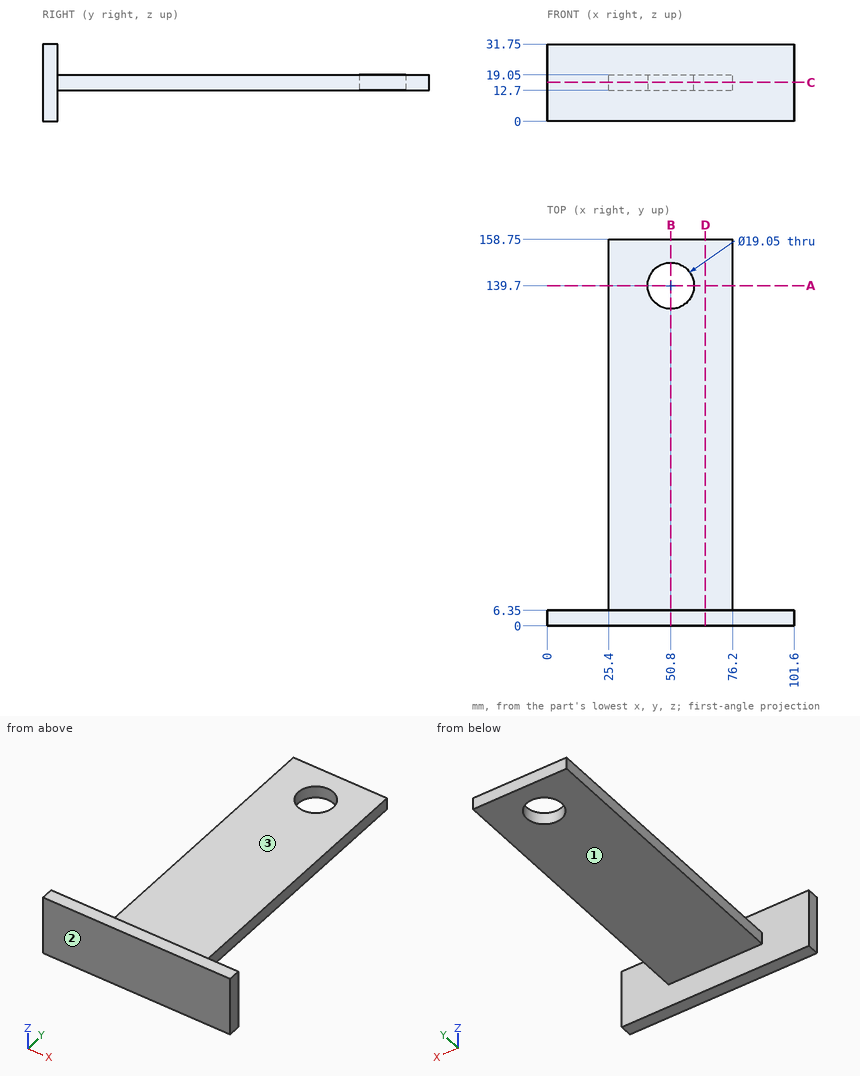
Source: three-view drawing plus pictorial views. Frame: mm from the lowest corner of the part. A direction names the side the tool comes from. Round coordinates to 2 decimals unless told otherwise and drop trailing zeros. Order: outer loops, then holes, each group sorted by start corner. A loop starts at its lowest first (then second) coordinate and runs counter-clockwise, first axis right, second up. Notation, with made-up numbers: (11, 44) -> (70, 44) arc R19 ccw to (70, 63) -> close; hole circle Ø6 at (26.5, -9.5). An arc over 180 degrees is marked (long way). Use CSV: the item, a comma, the result in double quotes. Start each with the question number.
1) Section C-C (z = 16). Return the cut outline in (x, y) (3 decimals).
2) Set-up query: the marked faces 1, 2 and 3. Return all of +Z, -Z, +X, -X, +Y, -Y with unobstructed straight access to the full face (end or side cutting, diameter ignored); none if empty.
3) Section B-B (x = 50.8). Return the cut outline in (y, z) (3 decimals).
4) Section A-A (y = 139.7). Return the cut outline in (x, z) (3 decimals), and give its area (3 significant figures).
5) Section D-D (x = 65). Return the cut outline in (y, z), and give its area (3 significant figures).
6) Material intervals for line 1 along Y through (x, z) = (50, 17); line 2 along X through (y, z) = (139.7, 17.75) (3 decimals); line 3 along Y through (x, z) = (20, 2.5), sorted ascending. Write a range as from..to.
7) First-contact query: pin 1 Ø6 at (x, y) = (63.5, 104) entering from +Z; pin 2 Ø3 at (y, z) = (84, 16) entering from +X; pin 3 Ø5 at (x, y) = (24.5, 117.5) entering from -Z; pin 4 Ø15 at (x, y) = (50.8, 139.7) entering from -Z. Flat tips, straight axial feed; report the tip coordinate or a pass-through.
Returned:
1,outline,"(0, 0) -> (101.6, 0) -> (101.6, 6.35) -> (76.2, 6.35) -> (76.2, 158.75) -> (25.4, 158.75) -> (25.4, 6.35) -> (0, 6.35) -> close; hole circle Ø19.05 at (50.8, 139.7)"
2,face 1,"-Z, +X, -X, +Y"
2,face 2,"+Z, -Z, +X, -X, -Y"
2,face 3,"+Z, +X, -X, +Y"
3,outline,"(0, 0) -> (6.35, 0) -> (6.35, 12.7) -> (130.175, 12.7) -> (130.175, 19.05) -> (6.35, 19.05) -> (6.35, 31.75) -> (0, 31.75) -> close; (149.225, 12.7) -> (158.75, 12.7) -> (158.75, 19.05) -> (149.225, 19.05) -> close"
4,outline,"(25.4, 12.7) -> (41.275, 12.7) -> (41.275, 19.05) -> (25.4, 19.05) -> close; (60.325, 12.7) -> (76.2, 12.7) -> (76.2, 19.05) -> (60.325, 19.05) -> close"
4,area,"202 mm²"
5,outline,"(0, 0) -> (6.35, 0) -> (6.35, 12.7) -> (158.75, 12.7) -> (158.75, 19.05) -> (6.35, 19.05) -> (6.35, 31.75) -> (0, 31.75) -> close"
5,area,"1,170 mm²"
6,line 1,"y = 0..130.21, 149.19..158.75"
6,line 2,"x = 25.4..41.275, 60.325..76.2"
6,line 3,"y = 0..6.35"
7,pin 1,"stops at z = 19.05"
7,pin 2,"stops at x = 76.2"
7,pin 3,"stops at z = 12.7"
7,pin 4,"passes through"
